```python
from build123d import *

# Parameters (mm, degrees)
F0_W     = 15.875
F0_H     = 15.875
F1_DEPTH = 20.6375
F3_DEPTH = 15.876
F5_DEPTH = 15.876
F8_ANGLE = 90


with BuildPart() as f1:
    # F0 (on Top) → F1 (new body)
    with BuildSketch(Plane.XY):
        Rectangle(F0_W, F0_H)
    extrude(amount=-F1_DEPTH)

    # F2 (on face) → F3 (cut, through all)
    with BuildSketch(Plane.XZ.offset(7.9375)):
        Polygon((7.9375, 0), (3.175, 0), (7.9375, -15.875), align=None)
    extrude(amount=-F3_DEPTH, mode=Mode.SUBTRACT)

    # F4 (on face) → F5 (cut, through all)
    with BuildSketch(Plane.XZ.offset(7.9375)):
        Polygon((7.9375, -20.6375), (7.9375, -15.875), (3.175, -20.6375), align=None)
    extrude(amount=-F5_DEPTH, mode=Mode.SUBTRACT)


with BuildPart() as f1_1:
    # F6: moved
    add(f1.part.moved(Location((-7.9375, 0, 0))))


with BuildPart() as f1_2:
    # F7: moved
    add(f1_1.part.moved(Location((0, 7.9375, 0))))


with BuildPart() as f1_3:
    # F8: moved
    add(f1_2.part.rotate(Axis((-10.31875, 0, 0), (-1, 0, 0)), F8_ANGLE))


solid = f1_3.part
```
Model file for the job. Use its own axes, mm. Give positions to 0.01 mm unless a question says otherwise; leave off trailing zeros. Loops run counter-clockwise (first coordinate to the right, second up) from the corner with the lowest first, then second, coordinate; pieces in that order, holes last. Notation, with made-up numbers: M 18.25,-27.5 L 27.25,-27.5 A26 ccw 27.25,-3.5 Z; hole C -35.75,4.5 d2. An arc over 180 degrees is marked long. Use one line per item in the form item = value.
Item 1: Slice it at C-C on x = -1. List the corners of the cut face in (y, z) (3 decimals).
Filled in:
outline = M -16.875,-15.875 L -12.542,-15.875 L -12.542,0 L -16.875,0 Z
Item 2: Slice it at A-A on z = -2.75. List the corners of the cut face in (x, y) (1 decimal), and give its area (3 significant figures).
Filled in:
outline = M -15.9,-20.6 L -4.8,-20.6 L 0,-15.9 L -4.8,0 L -15.9,0 Z
area = 278 mm^2
Item 3: Drill centre lines: L1, parallel to X at y = -10.25, z = -3 (1 decimal); L2, parallel to X at y = -6.25, z = -7.25 (1 decimal). Where is each one in solid material? Low to high.
Filled in:
L1 = -15.9 to -1.7
L2 = -15.9 to -2.9
Item 4: Slice it at B-B on y = -8.5. List the corners of the cut face in (x, z) (1 decimal), and give its area (3 significant figures).
Filled in:
outline = M -15.9,-15.9 L -2.2,-15.9 L -2.2,0 L -15.9,0 Z
area = 217 mm^2
